Here's how the part is built. I have some questions about the finished solid (model axes, mm). A direction names the side the tool comes from. Coordinates: 2 decimals unless noted, no trailing zeros. Write each loop counter-clockwise with the first axis right and the second up, starting at its lowest first coordinate (ties: lowest second). Pieces come first, ordered by that corner, then holes.
Item 1: Please list where these lines run through material, in increasing order: line 1 (Y direction, x = 0, z = 2.35); line 2 (Y direction, x = -1, z = 1.25); line 3 (X direction, y = -17, z = 1.2).
Item 2: I want a section at C-C (z = 0.8). Count the separate pieces of the cut face and the enclosed holes in it, and give its area (3 significant figures).
Item 3: I want a section at D-D (x = 25). Please give me the cut outline in (y, z), and give its area (3 significant figures).
Item 4: For faces 4 (the face through (33.175, -20.814, 1.479)), 5 (the face through (20.492, 13.655, 1.479)), which set-ups out of +Z, -Z, +X, -X, +Y, -Y let a thin tool reach every point of the face, with its end or its side?
Item 5: I'm going to push a flat-ended pin straight in: P1, Ø3, axis at x = -5.66, y = -5.66, coming from the -Z side. Where does the tip first touch, or does it pass through?
Item 6: I want a section at A-A (x = 0). Please give me the cut outline in (y, z).
Item 7: If we mould it in two halves opening along Y, with no side actions, what happens to faces 1 (the face through (35, 0, 3)), 2 (the face through (45, 20, 1)), 3 (the face through (-0.867, -3.905, 1.479))? For each: pulls with the +Y half, pulls with the -Y half, needs draft (parallel to the pull), parting line crosses it, or undercut.
Item 8: I want a section at B-B (y = 0). Please give me the cut outline in (x, z).
from build123d import *

# Parameters (mm, degrees)
F0_R     = 4
F0_R_2   = 1.55
F1_DEPTH = 3


with BuildPart() as f1:
    # F0 (on Top) → F1 (new body)
    with BuildSketch(Plane.XY):
        with BuildLine():
            ThreePointArc((19.031669, 23.657734), (12.5, 20), (5.968331, 23.657734))
            ThreePointArc((5.968331, 23.657734), (-0.374988, 26.989949), (-6.325402, 22.998215))
            ThreePointArc((-6.325402, 22.998215), (-11.5, 0), (-6.325402, -22.998215))
            ThreePointArc((-6.325402, -22.998215), (-0.374988, -26.989949), (5.968331, -23.657734))
            ThreePointArc((5.968331, -23.657734), (12.5, -20), (19.031669, -23.657734))
            ThreePointArc((19.031669, -23.657734), (25.419903, -26.987394), (31.363415, -22.916667))
            ThreePointArc((31.363415, -22.916667), (33.208403, -20.791873), (35.908712, -20))
            Line((35.908712, -20), (53, -20))
            Line((53, -20), (53, 20))
            Line((53, 20), (35.908712, 20))
            ThreePointArc((35.908712, 20), (33.208403, 20.791873), (31.363415, 22.916667))
            ThreePointArc((31.363415, 22.916667), (25.419903, 26.987394), (19.031669, 23.657734))
        make_face()
        with Locations((0, -20)):
            Circle(F0_R, mode=Mode.SUBTRACT)
        with Locations((-5.656854, -5.656854)):
            Circle(F0_R_2, mode=Mode.SUBTRACT)
        with Locations((5.656854, -5.656854)):
            Circle(F0_R_2, mode=Mode.SUBTRACT)
        with Locations((25, -20)):
            Circle(F0_R, mode=Mode.SUBTRACT)
        with Locations((-5.656854, 5.656854)):
            Circle(F0_R_2, mode=Mode.SUBTRACT)
        Circle(F0_R, mode=Mode.SUBTRACT)
        with Locations((5.656854, 5.656854)):
            Circle(F0_R_2, mode=Mode.SUBTRACT)
        with BuildLine():
            ThreePointArc((13, 5.996174), (20.660714, 13.656888), (28.321429, 5.996174))
            Line((28.321429, 5.996174), (28.321429, -5.996174))
            ThreePointArc((28.321429, -5.996174), (20.660714, -13.656888), (13, -5.996174))
            Line((13, -5.996174), (13, 5.996174))
        make_face(mode=Mode.SUBTRACT)
        with Locations((0, 20)):
            Circle(F0_R, mode=Mode.SUBTRACT)
        with Locations((25, 20)):
            Circle(F0_R, mode=Mode.SUBTRACT)
    extrude(amount=F1_DEPTH)


solid = f1.part
Answer:
1. line 1: y = -27 to -24, -16 to -4, 4 to 16, 24 to 27
1. line 2: y = -26.93 to -23.87, -16.13 to -3.87, 3.87 to 16.13, 23.87 to 26.93
1. line 3: x = -8.74 to -2.65, 2.65 to 22.35, 27.65 to 53
2. separate pieces: 1
2. enclosed holes: 10
2. area: 2,210 mm2
3. outline: (-27, 0) - (-24, 0) - (-24, 3) - (-27, 3) - close; (-16, 0) - (-12.31, 0) - (-12.31, 3) - (-16, 3) - close; (12.31, 0) - (16, 0) - (16, 3) - (12.31, 3) - close; (24, 0) - (27, 0) - (27, 3) - (24, 3) - close
3. area: 40.1 mm2
4. face 4: +Z, -Z, +X, -Y
4. face 5: +Z, -Z
5. P1: passes through
6. outline: (-27, 0) - (-24, 0) - (-24, 3) - (-27, 3) - close; (-16, 0) - (-4, 0) - (-4, 3) - (-16, 3) - close; (4, 0) - (16, 0) - (16, 3) - (4, 3) - close; (24, 0) - (27, 0) - (27, 3) - (24, 3) - close
7. face 1: needs draft
7. face 2: pulls with the +Y half
7. face 3: undercut
8. outline: (-11.5, 0) - (-4, 0) - (-4, 3) - (-11.5, 3) - close; (4, 0) - (13, 0) - (13, 3) - (4, 3) - close; (28.32, 0) - (53, 0) - (53, 3) - (28.32, 3) - close
